Geometry check sheet. Reference: the model listing, model coordinates, mm. Coordinates: 2 decimals unless noted, no trailing zeros. Loops run counter-clockwise (first coordinate to the right, second up) from the corner with the lowest first, then second, coordinate; pieces in that order, holes last.
Autodesk Inventor part; units mm, degrees
ref_plane "YZ Plane" through (0, 0, 0) normal (1, 0, 0) x (0, 1, 0)
ref_plane "XZ Plane" through (0, 0, 0) normal (0, 1, 0) x (-1, 0, 0)
ref_plane "XY Plane" through (0, 0, 0) normal (0, 0, 1) x (1, 0, 0)
sketch "Sketch1" plane through (0, 0, 0) normal (0, 1, 0) x (-1, 0, 0)
  circle A0 centre (0, 0) radius 11.1125
  circle A1 centre (0, 0) radius 8 construction
  line L0 (0, 0) -> (0, -8) construction
  line L1 (0, 0) -> (5.6569, -5.6569) construction
  circle A2 centre (5.6569, -5.6569) radius 1.5
  circle A3 centre (-5.6569, 5.6569) radius 1.5
  circle A4 centre (0, 0) radius 5.25
  circle A5 centre (0, 0) radius 7.9375 construction
  line L2 (0, 0) -> (-5.6127, -5.6127) construction
  circle A6 centre (-5.6127, -5.6127) radius 1.5875
  circle A7 centre (5.6127, 5.6127) radius 1.5875
  dimension "d21" = 15.875
  dimension "d0" = 22.225
  dimension "d1" = 16
  dimension "d2" = 45
  dimension "d3" = 3
  dimension "d6" = 360
  dimension "d8" = 10.5
  dimension "d22" = 3.175
  dimension "d25" = 360
extrude "Extrusion1" add sketch "Sketch1" along normal blind 10
sketch "Sketch2" plane through (0, 0, 0) normal (1, 0, 0) x (0, 1, 0)
  line L0 (10, -11.1125) -> (10, 11.1125)
  line L1 (10, 0) -> (0, 0) construction
  circle A0 centre (6.5, 0) radius 2
  line L2 (0, -11.1125) -> (0, 11.1125)
  dimension "d11" = 4
  dimension "d12" = 6.5
extrude "Extrusion2" cut sketch "Sketch2" along normal through all both and the other way through all
chamfer "Chamfer1" distance 0.5 angle 45 2 edges at (5.25, 0, 0) (5.25, 10, 0)
chamfer "Chamfer2" distance 0.5 angle 45 2 edges at (11.1125, 10, 0) (11.1125, 0, 0)
chamfer "Chamfer3" distance 0.25 angle 45 3 edges at (-4.8541, 6.5004, 2) (-4.8541, 6.4996, -2) (5.25, 4.5, 0.0002)
properties part number "Hub Adapter" material "Nylon 6/6"
(1) Gauge pin test, flat ends, axial feed: pin 1 Ø2 at (y, z) = (1, -3.5) entering from +X; pin 2 Ø5 at (x, y) = (8, 6) entering from +Z; pin 3 Ø2.5 at (x, z) = (-5.66, -5.66) entering from -Y; pin 4 Ø2 at (y, z) = (6, -2.5) entering from +X. Record the tip position at first contact, or that the pin passes through.
Findings:
pin 1: stops at x = 10.83
pin 2: stops at z = 9.66
pin 3: passes through
pin 4: stops at x = 10.98
(2) Sectioned sample at A-A on x = 0. Record the cut outline in (y, z).
Findings:
outline: (0, -10.61) - (0.5, -11.11) - (9.5, -11.11) - (10, -10.61) - (10, -5.75) - (9.5, -5.25) - (0.5, -5.25) - (0, -5.75) - close; (0, 5.75) - (0.5, 5.25) - (9.5, 5.25) - (10, 5.75) - (10, 10.61) - (9.5, 11.11) - (0.5, 11.11) - (0, 10.61) - close
(3) Sectioned sample at B-B on y = 2. State how many separate pieces and enclosed holes the cut face has, and give its area (3 significant figures).
Findings:
separate pieces: 1
enclosed holes: 5
area: 271 mm2
(4) Scan lines: L1, parallel to X at y = 3.25, z = 0; L2, parallel to Y at x = -10, z = 0; L3, parallel to X at y = 7, z = -6.75. Record each from-to range of solid material in increasing order.
Findings:
L1: x = -11.11 to -5.25, 5.25 to 11.11
L2: y = 0 to 4.5, 8.5 to 10
L3: x = -8.83 to -6.68, -4.63 to 4.51, 6.72 to 8.83
(5) Draft check along Z on faces 1 (the flat face through (0, 0, -7)), 2 (the cylindrical face through (4.851, 4.93, 4.392)), 3 (the cylindrical face through (-10.6, 4.94, -3.34)). Enter one of: +Z half, -Z half, draft (parallel to the pull), parting line (faces both ways), or undercut.
Findings:
face 1: draft
face 2: undercut
face 3: parting line
